Solid Edge part; units mm, degrees
sketch "Sketch1" plane through (0, 0, 0) normal (0, -1, 0) x (1, 0, 0)
  line L0 (-8, 10) -> (-8, 19.5)
  line L1 (-8, 19.5) -> (-6, 19.5)
  line L2 (-6, 19.5) -> (-1.3, 15.4801)
  arc A0 (-1.3, 15.4801) -> (0, 15) centre (0, 17) ccw
  line L3 (0, 15) -> (0, 10)
  line L4 (0, 10) -> (-8, 10)
revolve "RevolvedProtrusion1" add sketch "Sketch1" angle 360 about axis through (-60, 0, 0) along (1, 0, 0)
mirror "Mirror1" about plane through (0, 0, 0) normal (1, 0, 0) of "RevolvedProtrusion1"
sketch "Sketch2" plane through (-8, 0, 0) normal (-1, 0, 0) x (0, -1, 0)
  circle A0 centre (0, 0) radius 12
extrude "Cutout1" cut sketch "Sketch2" against normal blind 11.5
chamfer "Fase_1" distance 0.5 angle 45 1 edges at (-8, 12, 0)
properties material "Aluminium, 1060"
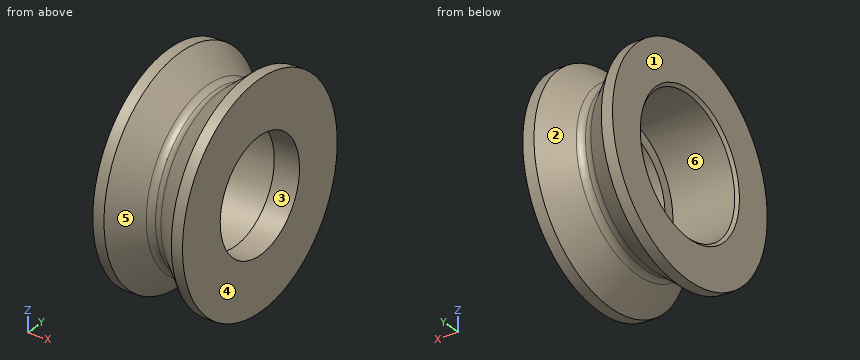
Verification items for the finished model (mm, model axes). Face numbers are marked on the shaded views. A direction names the side the tool comes from. Coordinates: 2 decimals unless noted, no trailing zeros. Order: outer loops, then holes, each group sorted by start corner. A loop starts at its lowest first (then second) coordinate and runs counter-clockwise, first axis right, second up. Notation, with made-up numbers: (82.5, -36) - (112.5, -36) arc R11 cw to (112.5, -19) - close; hole circle Ø10 at (25, 50.25). An arc over 180 degrees is marked (long way). Return JSON: item names as keys, results as strings.
(1) Access from +Z, -Z, +X, -X, +Y, -Y to the whole of each face (thin tool, end or side, straight path). Record for the marked faces 4, 5 and 6.
Filled sheet:
{"face 4": "+Z, -Z, +X, +Y, -Y", "face 5": "none", "face 6": "-X"}
(2) Section check D-D, the plane x = -2. Record the cut outline in (y, z), and give its area (3 significant figures).
Filled sheet:
{"outline": "circle Ø32.16 at (0, 0); hole circle Ø24 at (0, 0)", "area": "360 mm^2"}
(3) Section check A-A, the plane z = 0. Record the cut outline in (x, y).
Filled sheet:
{"outline": "(-8, -19.5) - (-6, -19.5) - (-1.3, -15.48) arc R2 cw to (1.3, -15.48) - (6, -19.5) - (8, -19.5) - (8, -10) - (3.5, -10) - (3.5, -12) - (-7.5, -12) - (-8, -12.5) - close; (-8, 12.5) - (-7.5, 12) - (3.5, 12) - (3.5, 10) - (8, 10) - (8, 19.5) - (6, 19.5) - (1.3, 15.48) arc R2 cw to (-1.3, 15.48) - (-6, 19.5) - (-8, 19.5) - close"}
(4) Section check C-C, the plane x = 5.5. Record the cut outline in (y, z), and give its area (3 significant figures).
Filled sheet:
{"outline": "circle Ø38.14 at (0, 0); hole circle Ø20 at (0, 0)", "area": "829 mm^2"}
(5) Go/stop test with flat-tipped pins: pin 1 (1.5 mm diameter, centred on x = 0, y = -1, fed in from +Z); pin 2 (8 mm diameter, centred on x = 5, y = 2.5, fed in from +Z); pin 3 (3 mm diameter, centred on y = 5.5, z = 9, fed in from -X); pin 4 (1 mm diameter, centred on x = 3.5, z = 2.5, fed in from +Y). Record where each tip stops, or that it passes through.
Filled sheet:
{"pin 1": "stops at z = 15.12", "pin 2": "stops at z = 19.5", "pin 3": "stops at x = -7.55", "pin 4": "stops at y = 17.62"}
(6) Thickness scan on line 1 along X through (y, z) = (14, 8.5); line 2 along Z through (x, y) = (1, 0); line 3 along Y through (x, z) = (-5, 7). Record the ranges inside material, lowest first.
Filled sheet:
{"line 1": "x = -8 to -2.35, 2.35 to 8", "line 2": "z = -15.27 to -12, 12 to 15.27", "line 3": "y = -17.28 to -9.75, 9.75 to 17.28"}
(7) Mould release check, pull along Z, two halves, no side actions. Record for the marked faces 1, 2 and 3: pulls with the +Z half, pulls with the -Z half, needs draft (parallel to the pull), parting line crosses it, or undercut.
Filled sheet:
{"face 1": "needs draft", "face 2": "parting line crosses it", "face 3": "undercut"}
